Here's how the part is built. I have some questions about the finished solid (model axes, mm). A direction names the side the tool comes from. Give positions to 0.01 mm unless a question says otherwise; leave off trailing zeros. Write each loop counter-clockwise with the first axis right and the second up, starting at its lowest first coordinate (ties: lowest second). Pieces come first, ordered by that corner, then holes. Notation, with made-up numbers: M 4,-10 L 48,-10 A20 cw 48,-5 Z; hole C 48,-35 d11. An arc over 180 degrees is marked long. Use one line per item in the form item = value. Start each with the question number.
from build123d import *

# Parameters (mm, degrees)
SKETCH1_R                = 2.55
BOSS_EXTRUDE1_DEPTH      = 5
SKETCH4_R                = 4.5
CUT_EXTRUDE2_DEPTH       = 1
SKETCH6_W                = 5.947651005
SKETCH6_H                = 20
BOSS_EXTRUDE2_DEPTH      = 4
BOSS_EXTRUDE2_DEPTH_BACK = 4
SKETCH11_R               = 4.5
CUT_EXTRUDE3_DEPTH       = 0.5
SKETCH16_R               = 3.25
BOSS_EXTRUDE3_DEPTH      = 3
BOSS_EXTRUDE3_DEPTH_BACK = 3
FILLET3_R                = 2
BOSS_EXTRUDE4_DEPTH      = 5.947651
CUT_EXTRUDE5_REACH       = 85
SKETCH18_R               = 3.25


with BuildPart() as part:
    # Sketch1 → Boss-Extrude1 (new body)
    with BuildSketch(Plane.XY):
        with BuildLine():
            Line((100, 25), (100, 20))
            ThreePointArc((100, 20), (99.414213562, 18.585786438), (98, 18))
            Line((98, 18), (72.248595461, 18))
            ThreePointArc((72.248595461, 18), (71.130561473, 17.658312395), (70.39454584, 16.75))
            ThreePointArc((70.39454584, 16.75), (50, 3), (29.60545416, 16.75))
            ThreePointArc((29.60545416, 16.75), (28.869438527, 17.658312395), (27.751404539, 18))
            Line((27.751404539, 18), (2, 18))
            ThreePointArc((2, 18), (0.585786438, 18.585786438), (0, 20))
            Line((0, 20), (0, 25))
            Line((0, 25), (0, 30))
            ThreePointArc((0, 30), (0.585786438, 31.414213562), (2, 32))
            Line((2, 32), (21.056240945, 32))
            Line((21.056240945, 32), (27.751404539, 32))
            ThreePointArc((27.751404539, 32), (28.869438527, 32.341687605), (29.60545416, 33.25))
            ThreePointArc((29.60545416, 33.25), (30.166752838, 34.520625347), (30.807119991, 35.753295167))
            ThreePointArc((30.807119991, 35.753295167), (32.106461975, 36.725482012), (33.699080137, 36.414026968))
            Line((33.699080137, 36.414026968), (35.34656276, 35.260447216))
            ThreePointArc((35.34656276, 35.260447216), (36.146649881, 34.078494315), (35.955031011, 32.664127224))
            ThreePointArc((35.955031011, 32.664127224), (50, 9), (64.044968989, 32.664127224))
            ThreePointArc((64.044968989, 32.664127224), (63.853350119, 34.078494315), (64.65343724, 35.260447216))
            Line((64.65343724, 35.260447216), (66.300919863, 36.414026968))
            ThreePointArc((66.300919863, 36.414026968), (67.893538025, 36.725482012), (69.192880009, 35.753295167))
            ThreePointArc((69.192880009, 35.753295167), (69.833247162, 34.520625347), (70.39454584, 33.25))
            ThreePointArc((70.39454584, 33.25), (71.130561473, 32.341687605), (72.248595461, 32))
            Line((72.248595461, 32), (78.943759055, 32))
            Line((78.943759055, 32), (98, 32))
            ThreePointArc((98, 32), (99.414213562, 31.414213562), (100, 30))
            Line((100, 30), (100, 25))
        make_face()
        with Locations((93, 25)):
            Circle(SKETCH1_R, mode=Mode.SUBTRACT)
        with Locations((7, 25)):
            Circle(SKETCH1_R, mode=Mode.SUBTRACT)
    extrude(amount=BOSS_EXTRUDE1_DEPTH)

    # Sketch4 → Cut-Extrude2 (cut)
    with BuildSketch(Plane.XY.offset(5)):
        with Locations((93, 25)):
            Circle(SKETCH4_R)
        with Locations((7, 25)):
            Circle(SKETCH4_R)
    extrude(amount=-CUT_EXTRUDE2_DEPTH, mode=Mode.SUBTRACT)

    # Sketch6 → Boss-Extrude2 (add, two sides)
    with BuildSketch(Plane(origin=(0, 25, 0), x_dir=(-1, 0, 0), z_dir=(0, -1, 0))) as boss_extrude2_sk:
        with Locations((-80.026174497, -15)):
            Rectangle(SKETCH6_W, SKETCH6_H)
    extrude(amount=BOSS_EXTRUDE2_DEPTH)
    extrude(boss_extrude2_sk.sketch, amount=-BOSS_EXTRUDE2_DEPTH_BACK)

    # Sketch11 → Cut-Extrude3 (cut)
    with BuildSketch(Plane(origin=(0, 0, 0), x_dir=(-1, 0, 0), z_dir=(0, 0, -1))):
        with Locations((-93, 25)):
            Circle(SKETCH11_R)
        with Locations((-7, 25)):
            Circle(SKETCH11_R)
    extrude(amount=-CUT_EXTRUDE3_DEPTH, mode=Mode.SUBTRACT)

    # Sketch16 → Boss-Extrude3 (add, two sides)
    with BuildSketch(Plane(origin=(0, 25, 0), x_dir=(-1, 0, 0), z_dir=(0, -1, 0))) as boss_extrude3_sk:
        with BuildLine():
            Line((-30.494270905, -5), (-22.494270905, -5))
            Line((-22.494270905, -5), (-22.494270905, -71))
            ThreePointArc((-22.494270905, -71), (-23.665843781, -73.828427125), (-26.494270905, -75))
            Line((-26.494270905, -75), (-30.494270905, -75))
            Line((-30.494270905, -75), (-47.361403242, -75))
            ThreePointArc((-47.361403242, -75), (-57.917236977, -76.464101615), (-53.018257491, -67))
            Line((-53.018257491, -67), (-34.494270905, -67))
            ThreePointArc((-34.494270905, -67), (-31.665843781, -65.828427125), (-30.494270905, -63))
            Line((-30.494270905, -63), (-30.494270905, -60.732138804))
            Line((-30.494270905, -60.732138804), (-47.361403242, -60.732138804))
            ThreePointArc((-47.361403242, -60.732138804), (-57.917236977, -62.196240419), (-53.018257491, -52.732138804))
            Line((-53.018257491, -52.732138804), (-34.494270905, -52.732138804))
            ThreePointArc((-34.494270905, -52.732138804), (-31.665843781, -51.560565928), (-30.494270905, -48.732138804))
            Line((-30.494270905, -48.732138804), (-30.494270905, -5))
        make_face()
        with Locations((-53.018257491, -73)):
            Circle(SKETCH16_R, mode=Mode.SUBTRACT)
        with Locations((-53.018257491, -58.732138804)):
            Circle(SKETCH16_R, mode=Mode.SUBTRACT)
    extrude(amount=BOSS_EXTRUDE3_DEPTH)
    extrude(boss_extrude3_sk.sketch, amount=-BOSS_EXTRUDE3_DEPTH_BACK)

    # Fillet3
    fillet3_edges = [part.edges().sort_by_distance(p)[0] for p in [
        (83, 25, 5),
        (80.026174498, 29, 5),
        (77.052348995, 25, 5),
        (80.026174498, 21, 5),
        (30.494270905, 25, 5),
        (26.494270905, 28, 5),
        (22.494270905, 25, 5),
        (26.494270905, 22, 5),
    ]]
    fillet(fillet3_edges, radius=FILLET3_R)

    # Sketch17 → Boss-Extrude4 (add)
    with BuildSketch(Plane(origin=(83, 0, 0), x_dir=(0, 0, -1), z_dir=(1, 0, 0))):
        with BuildLine():
            ThreePointArc((-19.547210182, 27.503414308), (-31, 25), (-19.547210182, 22.496585692))
            ThreePointArc((-19.547210182, 22.496585692), (-8.094420363, 25), (-19.547210182, 27.503414308))
        make_face()
    extrude(amount=-BOSS_EXTRUDE4_DEPTH)

    # Sketch18 → Cut-Extrude5 (cut, up to next)
    with BuildSketch(Plane(origin=(83, 0, 0), x_dir=(0, 0, -1), z_dir=(1, 0, 0)), mode=Mode.PRIVATE) as cut_extrude5_sk1:
        with Locations((-25, 25)):
            Circle(SKETCH18_R)
    cut_extrude5_tool1 = extrude(cut_extrude5_sk1.sketch, amount=-CUT_EXTRUDE5_REACH, mode=Mode.PRIVATE) & part.part
    add(cut_extrude5_tool1.solids().sort_by_distance((83, 25, 25))[0], mode=Mode.SUBTRACT)
    # Sketch18 → Cut-Extrude5 (cut, up to next)
    with BuildSketch(Plane(origin=(83, 0, 0), x_dir=(0, 0, -1), z_dir=(1, 0, 0)), mode=Mode.PRIVATE) as cut_extrude5_sk2:
        with Locations((-14.094420363, 25)):
            Circle(SKETCH18_R)
    cut_extrude5_tool2 = extrude(cut_extrude5_sk2.sketch, amount=-CUT_EXTRUDE5_REACH, mode=Mode.PRIVATE) & part.part
    add(cut_extrude5_tool2.solids().sort_by_distance((83, 25, 14.09442))[0], mode=Mode.SUBTRACT)


solid = part.part
1) Please list where these lines run through material, in increasing order: line 1 (X direction, y = 25, z = 3.1); line 2 (Z direction, x = 69, y = 33.5); line 3 (Z direction, x = 30, y = 25.5).
2) Will these pins go through, and if not, where does the flat tip stop? P1, Ø2, axis at x = 80.5, z = 19.5, coming from the -Y side; P2, Ø4, axis at x = 79, y = 32.5, coming from the +Z side; P3, Ø5.5, axis at x = 93, y = 25, coming from the +Z side.
3) Suppose I cut it at D-D, the plane z = 73. List the corners of the cut face in (x, y) for me.
4) Suppose I cut it at B-B, the plane z = 25. List the corners of the cut face in (x, y) for me.
5) On a 3-axis mill with a long thin cutter (end or side, diameter ignored), from which of +Z, -Z, +X, -X, +Y, -Y can I reach the whole of each face in a straight line? I mean faces 1 (the face through (5, 23, 0.5)), 2 (the face through (85, 32, 2)), 3 (the face through (88.504, 25.198, 4.507)), 4 (the face through (30.494, 25, 28)), 5 (the face through (80.068, 23.022, 27.579)). Say none if no direction works.
6) Suppose I cut it at A-A, the plane x = 93. List the corners of the cut face in (y, z) for me.
7) Suppose I cut it at C-C, the plane x = 57.5. List the corners of the cut face in (y, z) for me.
8) Thinking about a two-plate mould opening in Y: for faces 6 (the face through (32.08, 36.72, 2.46)), 7 (the face through (83, 25, 19)), 8 (the face through (95, 23, 4)), which applies, released by +Y, released by -Y, zero draft, split by the parting line, or undercut?
Checks:
q1.line_1 = 0 to 4.45, 9.55 to 34, 66 to 90.45, 95.55 to 100
q1.line_2 = 0 to 5
q1.line_3 = 0 to 75
q2.P1 = 20.93
q2.P2 = 27.4
q2.P3 = 4
q3.outline = M 23.03,22 L 49.77,22 L 49.77,28 L 23.03,28 Z; M 56.27,22 L 59.02,22 L 59.02,28 L 56.27,28 Z
q4.outline = M 22.49,22 L 30.49,22 L 30.49,28 L 22.49,28 Z; M 77.05,19 L 83,19 L 83,21.75 L 77.05,21.75 Z; M 77.05,28.25 L 83,28.25 L 83,31 L 77.05,31 Z
q5.face_1 = -Z
q5.face_2 = +Z, -Z, +X, +Y
q5.face_3 = +Z
q5.face_4 = +Y, -Y
q5.face_5 = +X
q6.outline = M 18,0 L 20.5,0 L 20.5,0.5 L 22.45,0.5 L 22.45,4 L 20.5,4 L 20.5,5 L 18,5 Z; M 27.55,0.5 L 29.5,0.5 L 29.5,0 L 32,0 L 32,5 L 29.5,5 L 29.5,4 L 27.55,4 Z
q7.outline = M 4.32,0 L 10.87,0 L 10.87,5 L 4.32,5 Z; M 22,54.74 L 28,54.74 L 28,62.72 L 22,62.72 Z; M 22,69.01 L 28,69.01 L 28,76.99 L 22,76.99 Z
q8.face_6 = released by +Y
q8.face_7 = zero draft
q8.face_8 = undercut
